from build123d import *

# Parameters (mm, degrees)
F1_DEPTH  = 12
F3_DEPTH  = 4
F2_R      = 1.75
F4_DEPTH  = 25
F5_R      = 2
F8_DEPTH  = 25
F9_W      = 2
F9_H      = 26
F10_DEPTH = 7
F11_R     = 6
F12_R     = 1.99999


# Not quite as in the source:
# - a fillet or chamfer is up to 0.001 mm smaller than in the source, because OpenCascade refuses the exact size


with BuildPart() as f1:
    # F0 (on Top) → F1 (new body)
    with BuildSketch(Plane.XY):
        Polygon((2, 15.0915228184), (0, 15.0915228184), (0, 7.0915228184), (57.4, 7.0915228184), (57.4, -3.9084771816), (59.4, -3.9084771816), (59.4, 9.0915228184), (2, 9.0915228184), align=None)
    extrude(amount=F1_DEPTH)

    # F3 (add): a face of the model
    f3_faces = [f1.faces().sort_by_distance(p)[0] for p in [
        (2, 12.0915228184, 6),
    ]]
    extrude(f3_faces, amount=F3_DEPTH)

    # F2 (on face) → F4 (cut)
    with BuildSketch(Plane(origin=(0, 0, 0), x_dir=(0, -1, 0), z_dir=(-1, 0, 0))):
        with Locations((-12.0915228184, 6)):
            Circle(F2_R)
    extrude(amount=-F4_DEPTH, mode=Mode.SUBTRACT)

    # F5
    f5_edges = [f1.edges().sort_by_distance(p)[0] for p in [
        (3, 15.091523, 0),
        (3, 15.091523, 12),
    ]]
    fillet(f5_edges, radius=F5_R)

    # F6: F1 across face


with BuildPart() as f1_1:
    add(f1.part)
    add(f1.part.mirror(Plane(origin=(58.4, -3.9084771816, 6), x_dir=(1, 0, 0), z_dir=(0, -1, 0))))

    # F7 (on face) → F8 (cut)
    with BuildSketch(Plane.YZ.offset(59.4)):
        Polygon((-1.9084771816, 7.5), (-3.9084771816, 7.5), (-5.9084771816, 7.5), (-5.9084771816, 0), (-1.9084771816, 0), align=None)
    extrude(amount=-F8_DEPTH, mode=Mode.SUBTRACT)

    # F9 (on face) → F10 (join)
    with BuildSketch(Plane.XY.offset(12)):
        with Locations((58.4, -3.9084771816)):
            Rectangle(F9_W, F9_H)
    extrude(amount=F10_DEPTH)

    # F11
    f11_edges = [f1_1.edges().sort_by_distance(p)[0] for p in [
        (57.4, -15.908477, 12),
        (57.4, 8.091523, 12),
    ]]
    fillet(f11_edges, radius=F11_R)

    # F12 (radius 2 in the source; OpenCascade refuses exactly that, so slightly less here)
    f12_edges = [f1_1.edges().sort_by_distance(p)[0] for p in [
        (58.4, -1.908477, 7.5),
        (58.4, -5.908477, 7.5),
    ]]
    fillet(f12_edges, radius=F12_R)


solid = f1_1.part
Source: CAD feature listing. Evaluate the final solid. Frame: model axes, mm. A direction names the side the tool comes from. Round coordinates to 2 decimals unless told otherwise and drop trailing zeros. Loops run counter-clockwise (first coordinate to the right, second up) from the corner with the lowest first, then second, coordinate; pieces in that order, holes last. Notation, with made-up numbers: (2.25, 70.25) - (25.25, 70.25) arc R24 ccw to (25.25, 99.25) - close; hole circle Ø4 at (2.5, 2.5). An arc over 180 degrees is marked (long way). Write item = value, one per line. Start each with the question number.
Item 1: Section query A-A on x = 19. Output: boundary loops of the cut face in (y, z).
Item 2: Material intervals for line 1 (Y direction, x = 40.5, z = 6); line 2 (Z direction, x = 14, y = -16); line 3 (X direction, y = 7, z = 13.75), sorted ascending.
Item 3: First-contact query: pin 1 Ø9.5 at (x, z) = (35.5, 5.5) entering from +Y; pin 2 Ø6 at (x, y) = (31.5, -16.5) entering from +Z; pin 3 Ø9.5 at (x, z) = (26, 11.5) entering from -Y; pin 4 Ø5 at (y, z) = (-3, 5.5) entering from +X. Flat tips, straight axial feed; report the tip coordinate or a pass-through.
Item 4: Section query B-B on y = -19.5. Output: boundary loops of the cut face in (x, z).
Item 5: Section query C-C on z = 13.5. Output: boundary loops of the cut face in (x, y), plus the area to 3 significant figures.
Item 6: Section query D-D on y = 3. Output: boundary loops of the cut face in (x, z), plus the area to 3 significant figures.
Item 7: Reachability of faces 1 (the face through (58, -5.908, 3)), 2 (the face through (19.6, -16.5, 12)), 3 (the face through (6, -18.5, 4.6)) from +Z, -Z, +X, -X, +Y, -Y: full face, straight path, thin tool, end or side. Return the list, or none.
Results list:
q1.outline = (-16.91, 0) - (-14.91, 0) - (-14.91, 12) - (-16.91, 12) - close; (7.09, 0) - (9.09, 0) - (9.09, 12) - (7.09, 12) - close
q2.line_1 = -16.91 to -14.91, 7.09 to 9.09
q2.line_2 = 0 to 12
q2.line_3 = 57.4 to 59.4
q3.pin_1 = 9.09
q3.pin_2 = 12
q3.pin_3 = -16.91
q3.pin_4 = 59.4
q4.outline = (0, 0) - (6, 0) - (6, 4.3) - (0, 4.3) - close; (0, 7.7) - (6, 7.7) - (6, 12) - (0, 12) - close
q5.outline = (55.37, -16.91) - (59.4, -16.91) - (59.4, 9.09) - (55.37, 9.09) - (55.37, 7.09) - (57.4, 7.09) - (57.4, -14.91) - (55.37, -14.91) - close
q5.area = 60.1 mm²
q6.outline = (57.4, 0) - (59.4, 0) - (59.4, 19) - (57.4, 19) - close
q6.area = 38.0 mm²
q7.face_1 = -Z, +X, -X
q7.face_2 = +Z, -X, +Y, -Y
q7.face_3 = +Z, -Z, +X, -Y
